Could you check a few things on this model? Use its own coordinates, in mm. A direction names the side the tool comes from. Give positions to 0.01 mm unless a question says otherwise; leave off trailing zeros. Order: outer loops, then holes, each group sorted by start corner. A loop starts at its lowest first (then second) coordinate and runs counter-clockwise, first axis right, second up. Notation, with made-up numbers: M -35,-11.5 L 18,-11.5 A21 cw 18,14.5 Z; hole C -14.5,8.5 d8. An arc over 180 degrees is marked long. Use a Markdown table: item, result. Add a question column.
```python
from build123d import *

# Parameters (mm, degrees)
SKETCH1_R           = 3.75
SKETCH1_W           = 66
SKETCH1_H           = 66
BOSS_EXTRUDE1_DEPTH = 100
SKETCH2_R           = 6
CUT_EXTRUDE1_DEPTH  = 10
SKETCH4_R           = 10.278687008
CUT_EXTRUDE2_DEPTH  = 10


with BuildPart() as part:
    # Sketch1 → Boss-Extrude1 (new body)
    with BuildSketch(Plane(origin=(0, 0, 0), x_dir=(1, 0, 0), z_dir=(0, 1, 0))):
        with BuildLine():
            Line((-152, 77), (152, 77))
            ThreePointArc((152, 77), (229, 0), (152, -77))
            Line((152, -77), (-152, -77))
            ThreePointArc((-152, -77), (-229, 0), (-152, 77))
        make_face()
        with Locations(Location((-104.964953983, 0, 0), (0, 0, 270))):
            Circle(SKETCH1_R, mode=Mode.SUBTRACT)
        with Locations(Location((104.964953983, 0, 0), (0, 0, 90))):
            Circle(SKETCH1_R, mode=Mode.SUBTRACT)
        Polygon((-141.697585802, 75), (142.523809524, 75), (33, 35), (-33, 35), align=None, mode=Mode.SUBTRACT)
        Polygon((-142.523809524, -75), (142.523809524, -75), (33, -35), (-33, -35), align=None, mode=Mode.SUBTRACT)
        with BuildLine():
            Line((-35, 32.680752833), (-150, 75))
            ThreePointArc((-150, 75), (-225, 0), (-150, -75))
            Line((-150, -75), (-35, -33))
            Line((-35, -33), (-35, -20.501152441))
            Line((-35, -20.501152441), (-62.070194122, -20.501152441))
            ThreePointArc((-62.070194122, -20.501152441), (-152.507121318, 0), (-62.070194122, 20.501152441))
            Line((-62.070194122, 20.501152441), (-35, 20.501152441))
            Line((-35, 20.501152441), (-35, 32.680752833))
        make_face(mode=Mode.SUBTRACT)
        with BuildLine():
            Line((35, 33), (35, 20.501152441))
            Line((35, 20.501152441), (62.070194122, 20.501152441))
            ThreePointArc((62.070194122, 20.501152441), (152.507121318, 0), (62.070194122, -20.501152441))
            Line((62.070194122, -20.501152441), (35, -20.501152441))
            Line((35, -20.501152441), (35, -33))
            Line((35, -33), (150, -75))
            ThreePointArc((150, -75), (225, 0), (150, 75))
            Line((150, 75), (35, 33))
        make_face(mode=Mode.SUBTRACT)
        Rectangle(SKETCH1_W, SKETCH1_H, mode=Mode.SUBTRACT)
        with BuildLine():
            Line((-61.249343804, 18.686976792), (-35, 18.686976792))
            Line((-35, 18.686976792), (-35, -18.686976792))
            Line((-35, -18.686976792), (-61.249343804, -18.686976792))
            ThreePointArc((-61.249343804, -18.686976792), (-57.422786648, 0), (-61.249343804, 18.686976792))
        make_face(mode=Mode.SUBTRACT)
        with BuildLine():
            Line((61.249343804, -18.686976792), (35, -18.686976792))
            Line((35, -18.686976792), (35, 18.686976792))
            Line((35, 18.686976792), (61.249343804, 18.686976792))
            ThreePointArc((61.249343804, 18.686976792), (57.422786648, 0), (61.249343804, -18.686976792))
        make_face(mode=Mode.SUBTRACT)
        with BuildLine():
            Line((-150.496141158, 1), (-110.630261894, 1))
            ThreePointArc((-110.630261894, 1), (-104.964953983, 5.752887425), (-99.299646072, 1))
            Line((-99.299646072, 1), (-59.433766808, 1))
            ThreePointArc((-59.433766808, 1), (-104.964953983, 45.542167335), (-150.496141158, 1))
        make_face(mode=Mode.SUBTRACT)
        with BuildLine():
            Line((-150.496141158, -1), (-110.630261894, -1))
            ThreePointArc((-110.630261894, -1), (-104.964953983, -5.752887425), (-99.299646072, -1))
            Line((-99.299646072, -1), (-59.433766808, -1))
            ThreePointArc((-59.433766808, -1), (-104.964953983, -45.542167335), (-150.496141158, -1))
        make_face(mode=Mode.SUBTRACT)
        with BuildLine():
            Line((59.433766808, 1), (99.299646072, 1))
            ThreePointArc((99.299646072, 1), (104.964953983, 5.752887425), (110.630261894, 1))
            Line((110.630261894, 1), (150.496141158, 1))
            ThreePointArc((150.496141158, 1), (104.964953983, 45.542167335), (59.433766808, 1))
        make_face(mode=Mode.SUBTRACT)
        with BuildLine():
            Line((59.433766808, -1), (99.299646072, -1))
            ThreePointArc((99.299646072, -1), (104.964953983, -5.752887425), (110.630261894, -1))
            Line((110.630261894, -1), (150.496141158, -1))
            ThreePointArc((150.496141158, -1), (104.964953983, -45.542167335), (59.433766808, -1))
        make_face(mode=Mode.SUBTRACT)
    extrude(amount=BOSS_EXTRUDE1_DEPTH)

    # Sketch2 → Cut-Extrude1 (cut)
    with BuildSketch(Plane.XY.offset(77)):
        with Locations((4.813758286, 27.006971007)):
            Circle(SKETCH2_R)
        with Locations((104.813758286, 27.006971007)):
            Circle(SKETCH2_R)
        with Locations((-95.186241714, 27.006971007)):
            Circle(SKETCH2_R)
    extrude(amount=-CUT_EXTRUDE1_DEPTH, mode=Mode.SUBTRACT)

    # Sketch4 → Cut-Extrude2 (cut)
    with BuildSketch(Plane(origin=(0, 0, -77), x_dir=(-1, 0, 0), z_dir=(0, 0, -1))):
        with Locations((0, 27.1)):
            Circle(SKETCH4_R)
        with Locations((100, 27.1)):
            Circle(SKETCH4_R)
        with Locations((-100, 27.1)):
            Circle(SKETCH4_R)
    extrude(amount=-CUT_EXTRUDE2_DEPTH, mode=Mode.SUBTRACT)


solid = part.part
```
1) Suppose I cut it at C-C on x = -79.5. Please give me the cut outline in (y, z), and give its area (3 significant figures).
2) Please list where these lines run through material, in increasing order: line 1 (Z direction, x = 18.5, y = 58.5); line 2 (Z direction, x = 44.5, y = 50); line 3 (X direction, y = 9, z = 20). Write a range as from..to.
3) Suppose I cut it at B-B on x = 24.5. Please give me the cut outline in (y, z).
4) For faces 3 (the face through (0, 49, 35)), 4 (the face through (-89.73, 27.55, -76.01)), 5 (the face through (1.1, 100, -34.6)), which set-ups out of +Z, -Z, +X, -X, +Y, -Y let a thin tool reach every point of the face, with its end or its side?
5) For pin 1 (6 mm diameter, centred on y = 60, z = 28.5, fed in from -X) (3 decimals); pin 2 (15.5 mm diameter, centred on x = 4.81, y = 27.01, fed in from +Z); pin 3 (9.5 mm diameter, centred on x = 104.81, y = 27.01, fed in from -Z); pin 4 (1 mm diameter, centred on y = 70.5, z = -46, fed in from -X), each with a flat end and sliding along its axis, tell me the tip position at first contact or that it passes through.
6) We'd pull the mould along X, two halves only. Please class faces 1 (the face through (1.1, 0, -34.6)), 2 (the face through (3.51, 21.15, 76.01)): pulls with the +X half, pulls with the -X half, needs draft (parallel to the pull), parting line crosses it, or undercut.
7) Suppose I cut it at A-A on z = -12.5. Count the separate pieces of the cut face and the enclosed holes in it, and give its area (3 significant figures).
Values found:
| question | item | result |
|---|---|---|
| 1 | outline | M 0,-77 L 100,-77 L 100,-75 L 0,-75 Z; M 0,-52.11 L 100,-52.11 L 100,-49.06 L 0,-49.06 Z; M 0,-40.15 L 100,-40.15 L 100,-37.76 L 0,-37.76 Z; M 0,-1 L 100,-1 L 100,1 L 0,1 Z; M 0,37.76 L 100,37.76 L 100,40.15 L 0,40.15 Z; M 0,49.25 L 100,49.25 L 100,51.98 L 0,51.98 Z; M 0,75 L 100,75 L 100,77 L 0,77 Z |
| 1 | area | 1,660 mm^2 |
| 2 | line 1 | z = -77..-75, -35..-33, 33..35, 75..77 |
| 2 | line 2 | z = -77..-75, -39.2..-36.47, -20.5..-18.69, 18.69..20.5, 36.47..39.2, 75..77 |
| 2 | line 3 | x = -226.36..-222.28, -148.1..-145.88, -64.05..-33, 33..64.05, 145.88..148.1, 222.28..226.36 |
| 3 | outline | M 0,-77 L 100,-77 L 100,-75 L 0,-75 Z; M 0,-35 L 100,-35 L 100,-33 L 0,-33 Z; M 0,33 L 100,33 L 100,35 L 0,35 Z; M 0,75 L 100,75 L 100,77 L 0,77 Z |
| 4 | face 3 | +Y, -Y |
| 4 | face 4 | -Z |
| 4 | face 5 | +Z, -Z, +X, -X, +Y |
| 5 | pin 1 | stops at x = -224.655 |
| 5 | pin 2 | stops at z = 77 |
| 5 | pin 3 | stops at z = -62.96 |
| 5 | pin 4 | stops at x = -214.12 |
| 6 | face 1 | needs draft |
| 6 | face 2 | undercut |
| 7 | separate pieces | 8 |
| 7 | enclosed holes | 0 |
| 7 | area | 2,040 mm^2 |
